Check sheet for the drawn part. Datum: minimum x, y, z corner. Units: mm. A direction names the side the tool comes from. Round coordinates to 2 decimals unless told otherwise and drop trailing zeros. Loops run counter-clockwise (first coordinate to the right, second up) from the corner with the lowest first, then second, coordinate; pieces in that order, holes last. Notation, with made-up numbers: (57, 47) -> (112, 47) arc R32 cw to (112, 75) -> close; hole circle Ø5 at (-39, 37). An arc over 180 degrees is marked (long way). Return JSON: item names as keys, results as strings.
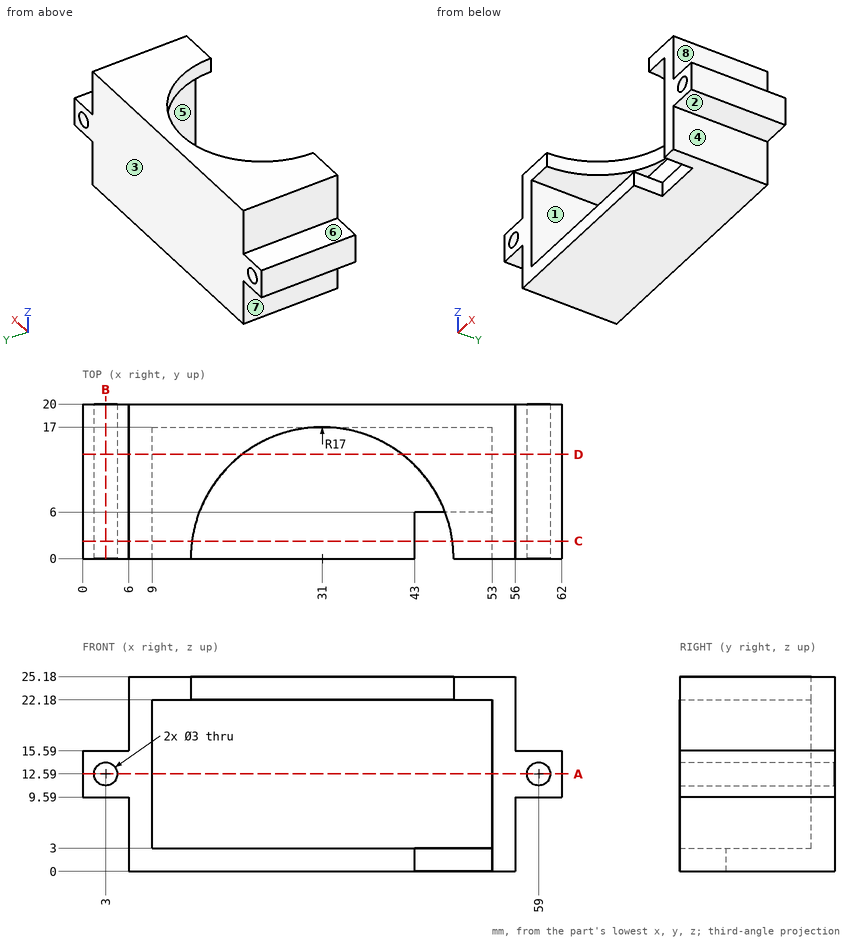
Q1. Go/stop test with flat-tipped pins: pin 1 (5 mm diameter, centred on x = 60, y = 7, fed in from -Z); pin 2 (3.5 mm diameter, centred on y = 2.5, z = 1.5, fed in from +X); pin 3 (8 mm diameter, centred on y = 4, z = 22.5, fed in from -X); pin 4 (2.5 mm diameter, centred on x = 3, z = 12.59, fed in from -Y). Record where each tip stops, or that it passes through.
Results list:
{"pin 1": "z = 9.59", "pin 2": "x = 56", "pin 3": "x = 6", "pin 4": "through"}
Q2. Draft check along Z on the marked faces 1, 2 and 3. Enter one of: released by +Z, released by -Z, zero draft, split by the parting line, or undercut.
Results list:
{"face 1": "undercut", "face 2": "released by -Z", "face 3": "zero draft"}
Q3. Section check B-B (x = 3). Record the boundary of the cut face in (y, z), then the cut area to 3 significant figures.
Results list:
{"outline": "(0, 9.59) -> (20, 9.59) -> (20, 11.09) -> (0, 11.09) -> close; (0, 14.09) -> (20, 14.09) -> (20, 15.59) -> (0, 15.59) -> close", "area": "60.0 mm^2"}
Q4. Material ranges on line 1 (X direction, y = 1, z = 12.75); line 2 (X direction, y = 2.25, z = 5.25); line 3 (X direction, y = 7.75, z = 15.25), recorded low to high.
Results list:
{"line 1": "0 to 1.51, 4.49 to 9, 53 to 57.51, 60.49 to 62", "line 2": "6 to 9, 53 to 56", "line 3": "0 to 9, 53 to 62"}
Q5. Section check D-D (y = 13.5). Record the boundary of the cut face in (x, z), then the cut area to 3 significant figures.
Results list:
{"outline": "(0, 9.59) -> (6, 9.59) -> (6, 0) -> (56, 0) -> (56, 9.59) -> (62, 9.59) -> (62, 15.59) -> (56, 15.59) -> (56, 25.18) -> (41.33, 25.18) -> (41.33, 22.18) -> (53, 22.18) -> (53, 3) -> (9, 3) -> (9, 22.18) -> (20.67, 22.18) -> (20.67, 25.18) -> (6, 25.18) -> (6, 15.59) -> (0, 15.59) -> close; hole circle Ø3 at (3, 12.59); hole circle Ø3 at (59, 12.59)", "area": "411 mm^2"}
Q6. Tool access check on the marked faces 4, 5, 6, 7 and 8. Record the directions out of +Z, -Z, +X, -X, +Y, -Y that give a thin tool (end or side, any length) a straight path to the whole face; none if there is none.
Results list:
{"face 4": "-Z, +X, +Y, -Y", "face 5": "-Y", "face 6": "+Z, -X, +Y, -Y", "face 7": "-Z, -X, +Y, -Y", "face 8": "+Z, +X, +Y, -Y"}
Q7. Section check C-C (y = 2.25). Record the boundary of the cut face in (x, z), then the cut area to 3 significant figures.
Results list:
{"outline": "(0, 9.59) -> (6, 9.59) -> (6, 0) -> (43, 0) -> (43, 3) -> (9, 3) -> (9, 22.18) -> (14.15, 22.18) -> (14.15, 25.18) -> (6, 25.18) -> (6, 15.59) -> (0, 15.59) -> close; (47.85, 22.18) -> (53, 22.18) -> (53, 0) -> (56, 0) -> (56, 9.59) -> (62, 9.59) -> (62, 15.59) -> (56, 15.59) -> (56, 25.18) -> (47.85, 25.18) -> close; hole circle Ø3 at (3, 12.59); hole circle Ø3 at (59, 12.59)", "area": "342 mm^2"}
Q8. Section check A-A (z = 12.59). Record the boundary of the cut face in (x, y).
Results list:
{"outline": "(0, 0) -> (1.5, 0) -> (1.5, 20) -> (0, 20) -> close; (4.5, 0) -> (9, 0) -> (9, 17) -> (53, 17) -> (53, 0) -> (57.5, 0) -> (57.5, 20) -> (4.5, 20) -> close; (60.5, 0) -> (62, 0) -> (62, 20) -> (60.5, 20) -> close"}
